Build history of the part. All positions in model axes, mm. A direction names the side the tool comes from. Give positions to 0.01 mm unless a question says otherwise; leave off trailing zeros. Loops run counter-clockwise (first coordinate to the right, second up) from the corner with the lowest first, then second, coordinate; pieces in that order, holes last.
1) Band-saw the part on A-A on z = 5.5. List the corners of the cut face in (x, y) (3 decimals), then the cut area to 3 significant figures.
2) Band-saw the part on D-D on z = 7.25. List the corners of the cut face in (x, y), then the cut area to 3 significant figures.
3) 3-axis set-ups, long thin cutter, end or side, ignore diameter. For faces 4 (the cylindrical face through (-7.493, 0.33, 0.74)), 5 (the flat face through (-3.025, 0, 2)): which of +Z, -Z, +X, -X, +Y, -Y reach the whole face in a straight line?
4) Wall check: line 1 (Y direction, x = 0, z = 7.8); line 2 (Y direction, x = -0.25, z = 1); line 3 (X direction, y = 0.5, z = 1.75) (3 decimals). Give the ranges that are in metal, low to high.
5) Flat gauge pins, fed straight in: P1, Ø1, axis at x = 4, z = 4, coming from the -Y side; P2, Ø1.6, axis at y = 0, z = 5, coming from the +X side; P3, Ø1.9, axis at x = 0, y = 0, coming from the -Z side. Where does each tip first touch, or does it go through?
6) Band-saw the part on C-C on z = 1.75. List the corners of the cut face in (x, y) (3 decimals), then the cut area to 3 significant figures.
7) Two-plate mould, pull along Y, no slides. Class faces 1 (the flat face through (0, -2, 11.5)), 2 (the cylindrical face through (-0.59, 4.46, 7.95)), 3 (the flat face through (-1.53, 2.61, 1.73)): +Y half, -Y half, draft (parallel to the pull), parting line (faces both ways), or undercut.
```python
from build123d import *

# Parameters (mm, degrees)
SKETCH_R        = 7.5
PAD_DEPTH       = 1.5
SKETCH001_R     = 4.5
PAD001_DEPTH    = 10
POCKET_DEPTH    = 6
SKETCH003_R     = 1.55
POCKET001_DEPTH = 11.501
POCKET002_DEPTH = 4
CHAMFER_SIZE    = 2.999
SKETCH005_R     = 1.55
PAD002_DEPTH    = 0.3
CHAMFER001_SIZE = 0.495


with BuildPart() as part:
    # Sketch → Pad (new body)
    with BuildSketch(Plane.XY):
        Circle(SKETCH_R)
    extrude(amount=PAD_DEPTH)

    # Sketch001 → Pad001 (new body)
    with BuildSketch(Plane.XY.offset(1.5)):
        Circle(SKETCH001_R)
    extrude(amount=PAD001_DEPTH)

    # Sketch002 → Pocket (cut)
    with BuildSketch(Plane(origin=(0, 0, 0), x_dir=(1, 0, 0), z_dir=(0, 0, -1))):
        Polygon((2.525, 1.457809), (0, 2.915619), (-2.525, 1.457809), (-2.525, -1.457809), (0, -2.915619), (2.525, -1.457809), align=None)
    extrude(amount=-POCKET_DEPTH, mode=Mode.SUBTRACT)

    # Sketch003 → Pocket001 (cut, through all)
    with BuildSketch(Plane.XY.offset(11.5)):
        Circle(SKETCH003_R)
    extrude(amount=-POCKET001_DEPTH, mode=Mode.SUBTRACT)

    # Sketch004 → Pocket002 (cut)
    with BuildSketch(Plane(origin=(0, 0, 0), x_dir=(1, 0, 0), z_dir=(0, 0, -1))):
        Polygon((3.025, 1.746485), (0, 3.492969), (-3.025, 1.746485), (-3.025, -1.746485), (0, -3.492969), (3.025, -1.746485), align=None)
    extrude(amount=-POCKET002_DEPTH, mode=Mode.SUBTRACT)

    # Chamfer
    chamfer_edges = [part.edges().sort_by_distance(p)[0] for p in [
        (-4.5, 0, 1.5),
    ]]
    chamfer(chamfer_edges, length=CHAMFER_SIZE)

    # Sketch005 → Pad002 (new body)
    with BuildSketch(Plane(origin=(0, 0, 6), x_dir=(1, 0, 0), z_dir=(0, 0, -1))):
        Circle(SKETCH005_R)
    extrude(amount=-PAD002_DEPTH)

    # Chamfer001
    chamfer001_edges = [part.edges().sort_by_distance(p)[0] for p in [
        (3.025, 0, 4),
        (1.5125, -2.619727, 4),
        (1.5125, 2.619727, 4),
        (-1.5125, -2.619727, 4),
        (-3.025, 0, 4),
        (-1.5125, 2.619727, 4),
    ]]
    chamfer(chamfer001_edges, length=CHAMFER001_SIZE)


solid = part.part
```
Findings below:
1. outline: circle Ø9 at (0, 0); hole (-2.525, -1.458) - (0, -2.916) - (2.525, -1.458) - (2.525, 1.458) - (0, 2.916) - (-2.525, 1.458) - close
1. area: 41.5 mm2
2. outline: circle Ø9 at (0, 0); hole circle Ø3.1 at (0, 0)
2. area: 56.1 mm2
3. face 4: +Z, -Z
3. face 5: -Z
4. line 1: y = -4.5 to -1.55, 1.55 to 4.5
4. line 2: y = -7.5 to -3.35, 3.35 to 7.5
4. line 3: x = -7.232 to -3.025, 3.025 to 7.232
5. P1: stops at y = -3.93
5. P2: stops at x = 4.8
5. P3: stops at z = 6
6. outline: circle Ø14.498 at (0, 0); hole (-3.025, -1.746) - (0, -3.493) - (3.025, -1.746) - (3.025, 1.746) - (0, 3.493) - (-3.025, 1.746) - close
6. area: 133 mm2
7. face 1: draft
7. face 2: parting line
7. face 3: undercut
